from build123d import *

# Parameters (mm, degrees)
F0_R       = 27.18
F1_DEPTH   = 910
F2_DEPTH   = 100
F3_SIZE2   = 100
F3_SIZE    = 27
F3_2_SIZE2 = 100
F3_2_SIZE  = 27
F3_3_SIZE2 = 100
F3_3_SIZE  = 27
F4_SIZE2   = 27
F4_SIZE    = 100


with BuildPart() as f1:
    # F0 (on Top) → F1 (new body)
    with BuildSketch(Plane.XY):
        with BuildLine():
            ThreePointArc((29.0890013579, -0.8), (29.0972502096, -0.4000378014), (29.1, 0))
            ThreePointArc((29.1, 0), (29.0972502096, 0.4000378014), (29.0890013579, 0.8))
            ThreePointArc((29.0890013579, 0.8), (14.55, 25.2013392501), (-13.8516803559, 25.5918141467))
            ThreePointArc((-13.8516803559, 25.5918141467), (-14.55, 25.2013392501), (-15.237321002, 24.7918141467))
            ThreePointArc((-15.237321002, 24.7918141467), (-29.1, 0), (-15.237321002, -24.7918141467))
            ThreePointArc((-15.237321002, -24.7918141467), (-14.55, -25.2013392501), (-13.8516803559, -25.5918141467))
            ThreePointArc((-13.8516803559, -25.5918141467), (14.55, -25.2013392501), (29.0890013579, -0.8))
        make_face()
        Circle(F0_R, mode=Mode.SUBTRACT)
    extrude(amount=F1_DEPTH)

    # F0 (on Top) → F2 (join)
    with BuildSketch(Plane.XY):
        with BuildLine():
            ThreePointArc((29.0890013579, 0.8), (29.0972502096, 0.4000378014), (29.1, 0))
            ThreePointArc((29.1, 0), (29.0972502096, -0.4000378014), (29.0890013579, -0.8))
            Line((29.0890013579, -0.8), (144.0890013579, -0.8))
            Line((144.0890013579, -0.8), (144.0890013579, 0.8))
            Line((144.0890013579, 0.8), (29.0890013579, 0.8))
        make_face()
        with BuildLine():
            Line((-71.3516803559, -125.1847355819), (-13.8516803559, -25.5918141467))
            ThreePointArc((-13.8516803559, -25.5918141467), (-14.55, -25.2013392501), (-15.237321002, -24.7918141467))
            Line((-15.237321002, -24.7918141467), (-72.737321002, -124.3847355819))
            Line((-72.737321002, -124.3847355819), (-71.3516803559, -125.1847355819))
        make_face()
        with BuildLine():
            ThreePointArc((-15.237321002, 24.7918141467), (-14.55, 25.2013392501), (-13.8516803559, 25.5918141467))
            Line((-13.8516803559, 25.5918141467), (-71.3516803559, 125.1847355819))
            Line((-71.3516803559, 125.1847355819), (-72.737321002, 124.3847355819))
            Line((-72.737321002, 124.3847355819), (-15.237321002, 24.7918141467))
        make_face()
    extrude(amount=F2_DEPTH)

    # F3
    f3_edges = [f1.edges().sort_by_distance(p)[0] for p in [
        (-72.044501, -124.784736, 100),
    ]]
    f3_side = f1.faces().sort_by_distance((-72.044501, -124.784736, 50))[0]
    chamfer(f3_edges, length=F3_SIZE, length2=F3_SIZE2, reference=f3_side)

    # F3#2
    f3_2_edges = [f1.edges().sort_by_distance(p)[0] for p in [
        (144.089001, 0, 100),
    ]]
    f3_2_side = f1.faces().sort_by_distance((144.089001, 0, 50))[0]
    chamfer(f3_2_edges, length=F3_2_SIZE, length2=F3_2_SIZE2, reference=f3_2_side)

    # F3#3
    f3_3_edges = [f1.edges().sort_by_distance(p)[0] for p in [
        (-72.044501, 124.784736, 100),
    ]]
    f3_3_side = f1.faces().sort_by_distance((-72.044501, 124.784736, 50))[0]
    chamfer(f3_3_edges, length=F3_3_SIZE, length2=F3_3_SIZE2, reference=f3_3_side)

    # F4
    f4_edges = [f1.edges().sort_by_distance(p)[0] for p in [
        (144.089001, 0, 0),
        (-72.044501, 124.784736, 0),
        (-72.044501, -124.784736, 0),
    ]]
    f4_side = f1.faces().sort_by_distance((-28.768792, 0, 0))[0]
    chamfer(f4_edges, length=F4_SIZE, length2=F4_SIZE2, reference=f4_side)


solid = f1.part
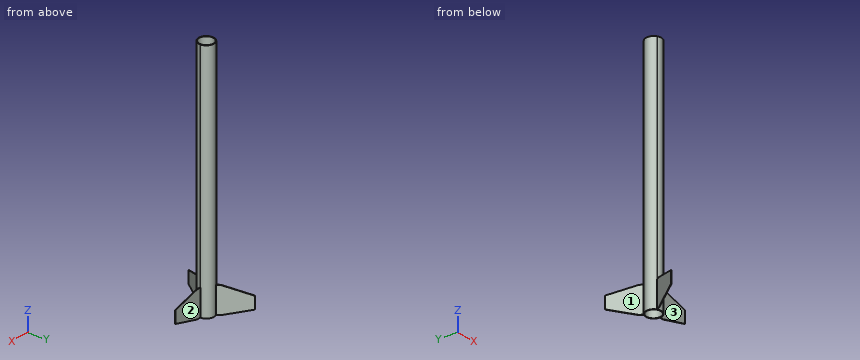
Work out the finished part from the listing and answer in its coordinate system (mm). Face numbers are marked on the shaded views. A direction names the side the tool comes from. Coordinates: 2 decimals unless noted, no trailing zeros. Write each loop counter-clockwise with the first axis right and the second up, starting at its lowest first coordinate (ties: lowest second). Pieces come first, ordered by that corner, then holes. Notation, with made-up numbers: M 86.5,51.5 L 102.5,51.5 A20 ccw 102.5,72.5 Z; hole C -21.75,-36 d10. An arc over 180 degrees is marked long. Use one line per item in the form item = value. Start each with the question number.
1. A tool of negligible diameter and unlimited length cuts with its end or side. For the marked faces 1, 2 and 3, from which of +Z, -Z, +X, -X, +Y, -Y can it reach the whole face along a straight path? Write none if from no direction.
2. Each of these flat-tipped pins is pushed along its axis until it touches: P1, Ø0.8, axis at x = 33, y = 0, coming from the +Z side; P2, Ø2, axis at x = 9, z = 332.5, coming from the +Y side; P3, Ø4, axis at x = -8, z = 428, coming from the +Y side; P4, Ø10, axis at y = -34.5, z = 150.5, coming from the +X side. Where does it stop, or does it pass through?
3. The part is cut by section C-C (x = 68.5). Give the vertices of the cut face in (y, z).
4. The part is cut by section D-D (y = -57.5). Give the vertices of the cut face in (x, z).
5. The part is cut by section A-A (x = 0). Give the vertices of the cut face in (y, z).
6. Straight lines are drawn through the part: probe 1 along Y at (x, z) = (0, 271); probe 2 along Y at (x, z) = (19, 530); probe 3 along X at (y, z) = (25, 611). For each, find the intervals that lie inside material, in ascending order. Write a range as from..to.
7. The part is cut by section B-B (z = 173.5). Give the vertices of the cut face in (x, y), plus the area to 3 significant figures.
Evaluation:
q1.face_1 = +Z, -Z, -X
q1.face_2 = +Z, -Z, +X, +Y
q1.face_3 = +Z, -Z, +X, -Y
q2.P1 = 100
q2.P2 = 27.98
q2.P3 = 28.47
q2.P4 = through
q3.outline = M -0.8,6.59 L 0.8,6.59 L 0.8,93.41 L -0.8,93.41 Z
q4.outline = M -34.12,6.15 L -32.27,5.9 L -32.27,94.1 L -34.12,93.85 Z
q5.outline = M -29.1,0 L -27.18,0 L -27.18,910 L -29.1,910 Z; M 27.18,0 L 29.1,0 L 29.1,910 L 27.18,910 Z
q6.probe_1 = -29.1..-27.18, 27.18..29.1
q6.probe_2 = -22.04..-19.44, 19.44..22.04
q6.probe_3 = -14.89..-10.67, 10.67..14.89
q7.outline = C 0,0 d58.2; hole C 0,0 d54.36
q7.area = 339 mm^2
